For this review, take the finished solid that the model builds, in its own axes (mm). A direction names the side the tool comes from. Give positions to 0.01 mm unless a question says otherwise; leave off trailing zeros. Write each loop counter-clockwise with the first axis right and the second up, starting at its lowest first coordinate (ties: lowest second). Pieces come first, ordered by that corner, then holes.
Q1. We need section A-A (y = 31.5). Write out the cut boundary in (x, z), then the cut area to 3 significant figures.
Q2. For line 1 (X direction, y = 48, z = 2); line 2 (X direction, y = 20.5, z = 3); line 3 (Z direction, x = 17, y = 59.5), list the stretches that pass through material, from the lowest coordinate up.
Q3. We need section B-B (x = 10). Write out the cut boundary in (y, z).
Q4. We need section C-C (x = -6). Write out the cut boundary in (y, z), then the cut area to 3 significant figures.
Q5. Machinability: for faces 5 (the flat face through (-3, 32, 4.946)), 6 (the cylindrical face through (10, 60.3, 2.4)), 7 (the flat face through (10.07, -9.86, 12.43)), which of the approach directions +Z, -Z, +X, -X, +Y, -Y give a long, thin tool a straight path to every point of the face, cutting with its end or side? Answer none if there is none.
Q6. We need section D-D (z = 14.5). Write out the cut boundary in (x, y), then the cut area to 3 significant figures.
Q7. Insertion check: P1, Ø1.5, axis at y = 37.5, z = 2, coming from the +X side; P2, Ø2, axis at x = -6, z = 16, coming from the +Y side; P3, Ø3, axis at x = -12, y = 38.5, coming from the +Z side. Each pin has a flat end and moves straight along its axis. Give the tip position at first contact, or say it passes through.
Q8. Mouldability with a two-part tool opening along X and no side actions: class faces 1 (the flat face through (-18.76, 22, 3)), 2 (the cylindrical face through (21.25, -9.86, 55.68)), 3 (the flat face through (-1.8, 33, 2)), 4 (the flat face through (23, 0, 5)) as released by +X, released by -X, zero draft, split by the parting line, or undercut.
```python
from build123d import *

# Parameters (mm, degrees)
CYLINDER004_R               = 1.8
CYLINDER004_DEPTH           = 10
BOX003_W                    = 3.6
BOX003_H                    = 50
BOX003_DEPTH                = 10
CYLINDER003_R               = 1.8
CYLINDER003_DEPTH           = 10
ARRAY001_X_COUNT            = 2
ARRAY001_X_PITCH            = 10
EXTRUDE005_DEPTH            = 65
CYLINDER002_R               = 2.2
CYLINDER002_DEPTH           = 20
CYLINDER002_PLACEMENT_ANGLE = 127.63
PAD_DEPTH                   = 20


with BuildPart() as cylinder004:
    # Cylinder004 → Cylinder004 (new body)
    with BuildSketch(Plane(origin=(0, 50, 0), x_dir=(1, 0, 0), z_dir=(0, 0, 1))):
        Circle(CYLINDER004_R)
    extrude(amount=CYLINDER004_DEPTH)


with BuildPart() as cube:
    # Box003 → Box003 (new body)
    with BuildSketch(Plane(origin=(-1.8, 0, 0), x_dir=(1, 0, 0), z_dir=(0, 0, 1))):
        with Locations((1.8, 25)):
            Rectangle(BOX003_W, BOX003_H)
    extrude(amount=BOX003_DEPTH)


with BuildPart() as array001:
    # Cylinder003 → Cylinder003 (new body)
    with BuildSketch(Plane.XY):
        Circle(CYLINDER003_R)
    extrude(amount=CYLINDER003_DEPTH)

    # Fusion004: union Cylinder004, Cube
    add(cylinder004.part)
    add(cube.part)

    # Array001 X: Array001 ×2


with BuildPart() as array001_1:
    add(array001.part)
    with Locations(*[(i * ARRAY001_X_PITCH, 0, 0) for i in range(1, ARRAY001_X_COUNT)]):
        add(array001.part)


with BuildPart() as array001_2:
    # Array001 placement: moved
    add(array001_1.part.moved(Location((0, 8.5, 0))))


with BuildPart() as cut002:
    # Sketch006 → Extrude005 (new body)
    with BuildSketch(Plane.XZ):
        Polygon((-18.759547, 0), (22.810035, 0), (19.860366, 4.945604), (-18.759547, 4.945604), align=None)
    extrude(amount=-EXTRUDE005_DEPTH)

    # Cut002: cut Array001
    add(array001_2.part, mode=Mode.SUBTRACT)


with BuildPart() as insert_hole:
    # Cylinder002 → Cylinder002 (new body)
    with BuildSketch(Plane.XY):
        Circle(CYLINDER002_R)
    extrude(amount=CYLINDER002_DEPTH)


with BuildPart() as insert_hole_1:
    # Cylinder002 placement: moved
    add(insert_hole.part.moved(Location((10.5, -10, 56.79))).rotate(Axis((10.5, -10, 56.79), (0, 1, 0)), CYLINDER002_PLACEMENT_ANGLE))


with BuildPart() as fusion003:
    # Sketch005 → Pad (new body)
    with BuildSketch(Plane.XZ):
        with BuildLine():
            Line((-18.759547, 0), (22.810035, 0))
            Line((22.810035, 0), (26.15983, 4.38135))
            ThreePointArc((26.15983, 4.38135), (26.531558, 5.778404), (25.806542, 7.029122))
            Line((25.806542, 7.029122), (24.559787, 7.982338))
            ThreePointArc((24.559787, 7.982338), (23.162733, 8.354066), (21.912015, 7.62905))
            Line((19.860366, 4.945604), (21.912015, 7.62905))
            Line((19.860366, 4.945604), (0, 20.13))
            Line((0, 20.13), (25.509785, 53.495414))
            Line((25.509785, 53.495414), (23.431531, 55.084359))
            ThreePointArc((23.431531, 55.084359), (21.212635, 55.674762), (19.22616, 54.523243))
            Line((-18.759547, 4.84), (19.22616, 54.523243))
            Line((-18.759547, 0), (-18.759547, 4.84))
        make_face()
    extrude(amount=PAD_DEPTH)

    # Cut: cut insert hole
    add(insert_hole_1.part, mode=Mode.SUBTRACT)

    # Fusion003: union Cut002
    add(cut002.part)


solid = fusion003.part
```
Computed:
1. outline: (-18.76, 0) - (-1.8, 0) - (-1.8, 4.95) - (-18.76, 4.95) - close; (1.8, 0) - (8.2, 0) - (8.2, 4.95) - (1.8, 4.95) - close; (11.8, 0) - (22.81, 0) - (19.86, 4.95) - (11.8, 4.95) - close
1. area: 163 mm2
2. line 1: x = -18.76 to -1.8, 1.8 to 8.2, 11.8 to 21.62
2. line 2: x = -18.76 to -1.8, 1.8 to 8.2, 11.8 to 21.02
2. line 3: z = 0 to 4.95
3. outline: (-20, 0) - (6.7, 0) - (6.7, 4.95) - (0, 4.95) - (0, 12.48) - (-20, 12.48) - close; (-20, 33.21) - (0, 33.21) - (0, 42.46) - (-20, 42.46) - close; (60.3, 0) - (65, 0) - (65, 4.95) - (60.3, 4.95) - close
4. outline: (-20, 0) - (65, 0) - (65, 4.95) - (0, 4.95) - (0, 21.53) - (-20, 21.53) - close
4. area: 752 mm2
5. face 5: +Z, +X, -X, +Y
5. face 6: +Z, -Z
5. face 7: +Y, -Y
6. outline: (-11.37, -20) - (7.36, -20) - (7.36, 0) - (-11.37, 0) - close
6. area: 375 mm2
7. P1: stops at x = 22.06
7. P2: stops at y = 0
7. P3: stops at z = 4.95
8. face 1: released by -X
8. face 2: split by the parting line
8. face 3: undercut
8. face 4: zero draft
